Design review of the part built by this model. Coordinates are the model's own, in mm. Coordinates: 2 decimals unless noted, no trailing zeros. Write each loop counter-clockwise with the first axis right and the second up, starting at its lowest first coordinate (ties: lowest second). Pieces come first, ordered by that corner, then holes.
Q1. Take a section at D-D (x = 91.5). Give the boundary of the cut face in (y, z), and give its area (3 significant figures).
Q2. Insertion check: pin 1 (1.5 mm diameter, centred on x = 64, z = -2.5, fed in from +Y); pin 2 (10 mm diameter, centred on x = 97, y = 1437.5, fed in from +Z). Each pin has a flat end and moves straight along its axis. Give the tip position at first contact, or say it passes through.
Q3. Take a section at C-C (z = -2.55). State how many separate pieces and enclosed holes the cut face has, and give its area (3 significant figures).
Q4. For probe 1 along X at (y, z) = (1444.75, -1.8); probe 2 along X at (y, z) = (1446, -0.9); probe 3 along X at (y, z) = (1439.25, -0.25), list the stretches that pass through material, from the lowest coordinate up.
Q5. Take a section at A-A (x = 67). Give the boundary of the cut face in (y, z).
Q6. Take a section at B-B (y = 1437.25). Give the boundary of the cut face in (x, z).
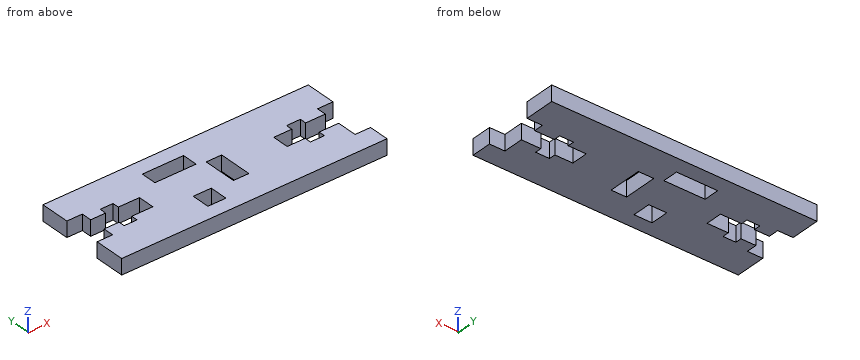
```python
from build123d import *

# Parameters (mm, degrees)
T_LE_DE_BASE_PLI_E1_DEPTH = 3


# Sheet-metal steps are written as plain solids
with BuildPart() as part:
    # Esquisse1 → Tôle de base pliée1 (new body)
    with BuildSketch(Plane.XY):
        Polygon((56.011486003, 1451.999694839), (107.511486003, 1451.228417484), (107.423076338, 1445.325096569), (104.423412714, 1445.370020309), (104.395809304, 1443.526875799), (100.595809304, 1443.583785584), (100.614677274, 1444.843644306), (97.914677274, 1444.884080206), (97.895809304, 1443.624221484), (94.395809304, 1443.676638392), (94.347885274, 1440.476638392), (97.847885274, 1440.424221484), (97.829017303, 1439.164362762), (100.529017303, 1439.123926862), (100.547885274, 1440.383785584), (104.347885274, 1440.326875799), (104.289178337, 1436.406875799), (107.289178337, 1436.361947021), (107.230300273, 1432.430520402), (55.729627521, 1433.201807832), (55.81730132, 1439.055993264), (58.81730132, 1439.011064486), (58.847926704, 1441.055993264), (61.74760154, 1441.012566982), (61.729288791, 1439.789781712), (64.228728196, 1439.752349459), (64.247596167, 1441.012208181), (68.347416735, 1440.950808205), (68.395340765, 1444.150808205), (64.295520197, 1444.212208181), (64.314426556, 1445.474630165), (61.814987151, 1445.512062418), (61.795520197, 1444.212208181), (58.89584536, 1444.255634463), (58.92579452, 1446.255410213), (55.926130896, 1446.300333953), align=None)
        Polygon((72.811486003, 1448.747757268), (80.811486003, 1448.627947194), (80.766562262, 1445.62828357), (72.766562262, 1445.748093644), align=None, mode=Mode.SUBTRACT)
        Polygon((82.316965577, 1445.105008259), (82.219630807, 1438.605737073), (85.219294431, 1438.560813333), (85.316629201, 1445.060084519), align=None, mode=Mode.SUBTRACT)
        Polygon((74.832038551, 1439.21643164), (78.332038551, 1439.164014732), (78.279627521, 1435.664407171), (74.779627521, 1435.716824078), align=None, mode=Mode.SUBTRACT)
    extrude(amount=-T_LE_DE_BASE_PLI_E1_DEPTH)


solid = part.part
```
Response:
1. outline: (1432.67, -3) - (1451.47, -3) - (1451.47, 0) - (1432.67, 0) - close
1. area: 56.4 mm2
2. pin 1: stops at y = 1451.89
2. pin 2: stops at z = 0
3. separate pieces: 1
3. enclosed holes: 3
3. area: 788 mm2
4. probe 1: x = 58.9 to 61.8, 64.3 to 82.31, 85.31 to 97.91, 100.61 to 104.41
4. probe 2: x = 58.92 to 72.77, 80.77 to 107.43
4. probe 3: x = 58.82 to 82.23, 85.23 to 97.83, 100.53 to 104.33
5. outline: (1433.03, -3) - (1440.97, -3) - (1440.97, 0) - (1433.03, 0) - close; (1444.17, -3) - (1451.84, -3) - (1451.84, 0) - (1444.17, 0) - close
6. outline: (55.79, -3) - (74.8, -3) - (74.8, 0) - (55.79, 0) - close; (78.3, -3) - (104.3, -3) - (104.3, 0) - (78.3, 0) - close
